from build123d import *

# Parameters (mm, degrees)
CHAMFER_1_SIZE           = 1
SKETCH_2_R               = 2.2
CUT_EXTRUDE_1_DEPTH      = 38.563279942
PATTERN_CIRCULAR_1_COUNT = 4


with BuildPart() as part:
    # Эскиз1 → Повернуть1 (revolve)
    with BuildSketch(Plane.XY, mode=Mode.PRIVATE) as revolve_1_sk:
        Polygon((0, -3.5), (0, -6), (6.2, -6), (6.2, -11), (8.2, -11), (8.2, -10.75), (12, -10.75), (12, -21), (18, -21), (18, -9), (35, -9), (35, -4.188), (25, -4.188), (22.582057073, 0), (19.020725942, 0), (17, -3.5), align=None)
    revolve(revolve_1_sk.sketch.rotate(Axis((0, 0, 0), (1, 0, 0)), 270), axis=Axis((0, 0, 0), (1, 0, 0)))

    # Фаска1
    chamfer_1_edges = [part.edges().sort_by_distance(p)[0] for p in [
        (35, 0, -4.188),
        (35, 0, -9),
    ]]
    chamfer(chamfer_1_edges, length=CHAMFER_1_SIZE)

    # Эскиз2 → Вырез-Вытянуть1 (cut, through all)
    with BuildSketch(Plane.ZY.offset(-12)):
        with Locations((0, 16)):
            Circle(SKETCH_2_R)
    cut_extrude_1 = extrude(amount=-CUT_EXTRUDE_1_DEPTH, mode=Mode.SUBTRACT)

    # Круговой массив1: Вырез-Вытянуть1 ×4 about axis
    pattern_circular_1_axis = Axis((0, 0, 0), (1, 0, 0))
    for i in range(1, PATTERN_CIRCULAR_1_COUNT):
        add(cut_extrude_1.rotate(pattern_circular_1_axis, i * 360 / PATTERN_CIRCULAR_1_COUNT), mode=Mode.SUBTRACT)


solid = part.part
CAD build for the part. Positions are in the model's coordinates, mm. A direction names the side the tool comes from. Give positions to 0.01 mm unless a question says otherwise; leave off trailing zeros. Write each loop counter-clockwise with the first axis right and the second up, starting at its lowest first coordinate (ties: lowest second). Pieces come first, ordered by that corner, then holes. Notation, with made-up numbers: (38, 88) - (66, 88) arc R19 cw to (66, 108) - close; hole circle Ø6 at (-16, -20). An arc over 180 degrees is marked (long way). Put each result on its own line as item: value.
(1) Saw through at D-D (x = 4). List the corners of the cut face in (y, z), then the cut area to 3 significant figures.
Working result:
outline: circle Ø12 at (0, 0); hole circle Ø7 at (0, 0)
area: 74.6 mm^2
(2) Wall check: L1, parallel to Y at x = 29, z = 0; L2, parallel to Y at x = 15, z = 0; L3, parallel to X at y = -18.5, z = 1.5. Give the ranges that are in metal, low to high.
Working result:
L1: -9 to -4.19, 4.19 to 9
L2: -21 to -18.2, -13.8 to -3.5, 3.5 to 13.8, 18.2 to 21
L3: 12 to 18
(3) Tool access for faces 1 (the cylindrical face through (10.13, -7.27, -7.92)), 2 (the cylindrical face through (3.143, -1.802, 5.723)), 3 (the cylindrical face through (14.958, -0.477, -13.852)), 4 (the cylindrical face through (29.437, -0.184, -4.184)), 5 (the flat face through (0, 3, -3)): list every direction of +Z, -Z, +X, -X, +Y, -Y with a clear straight run to the whole face (end or side of a thin tool).
Working result:
face 1: none
face 2: -X
face 3: +X, -X
face 4: +X
face 5: +Z, -Z, -X, +Y, -Y
(4) Saw through at B-B (z = 16). List the corners of the cut face in (x, y), then the cut area to 3 significant figures.
Working result:
outline: (12, -13.6) - (18, -13.6) - (18, -2.2) - (12, -2.2) - close; (12, 2.2) - (18, 2.2) - (18, 13.6) - (12, 13.6) - close
area: 137 mm^2
(5) Saw through at A-A (x = 13). List the corners of the cut face in (y, z).
Working result:
outline: circle Ø42 at (0, 0); hole circle Ø4.4 at (-16, 0); hole circle Ø7 at (0, 0); hole circle Ø4.4 at (0, -16); hole circle Ø4.4 at (0, 16); hole circle Ø4.4 at (16, 0)
(6) Pull direction Y, two halves, no side cores. Call faces 6 (the cylindrical face through (8.381, 3.417, -0.759)), 7 (the flat face through (6.2, 5, -5)), 8 (the cylindrical face through (15.04, -6.31, 20.03)): released by +Y, released by -Y, zero draft, split by the parting line, or undercut.
Working result:
face 6: undercut
face 7: zero draft
face 8: split by the parting line
(7) Drop flat-ended pins along their axis: pin 1 Ø4 at (y, z) = (3, 9.5) entering from -X; pin 2 Ø8 at (x, y) = (13.5, -15) entering from -Z; pin 3 Ø3 at (y, z) = (-16, 13.5) entering from +X. Give the stop position or say it passes through.
Working result:
pin 1: x = 6.2
pin 2: z = -17.89
pin 3: x = 18
